The listing builds one solid part. Answer for the finished solid, in the listing's coordinates (mm). Give positions to 0.01 mm unless a question says otherwise; leave off trailing zeros. Order: outer loops, then holes, each group sorted by start corner. A loop starts at its lowest first (then second) coordinate and runs counter-clockwise, first axis right, second up. Notation, with made-up numbers: (81, 44.5) -> (121, 44.5) arc R17 cw to (121, 67.5) -> close; hole circle Ø2 at (-36, -39). An arc over 180 degrees is marked (long way). Write item = value, one per line. Start each with the question number.
```python
from build123d import *

# Parameters (mm, degrees)
SALIENTE_EXTRUIR1_DEPTH = 3
CROQUIS2_W              = 3
CROQUIS2_H              = 16
CROQUIS2_H_2            = 15
SALIENTE_EXTRUIR2_DEPTH = 3


with BuildPart() as part:
    # Croquis1 → Saliente-Extruir1 (new body)
    with BuildSketch(Plane.XY):
        Polygon((111, -25), (-111, -25), (-111, -1.5), (-108, -1.5), (-108, -3), (-105, -3), (-105, 3), (-108, 3), (-108, 1.5), (-111, 1.5), (-111, 25), (111, 25), (111, 1.5), (108, 1.5), (108, 3), (105, 3), (105, -3), (108, -3), (108, -1.5), (111, -1.5), align=None)
        with BuildLine():
            Line((80, -15), (-80, -15))
            ThreePointArc((-80, -15), (-95, 0), (-80, 15))
            Line((-80, 15), (80, 15))
            ThreePointArc((80, 15), (95, 0), (80, -15))
        make_face(mode=Mode.SUBTRACT)
    extrude(amount=SALIENTE_EXTRUIR1_DEPTH)

    # Croquis2 → Saliente-Extruir2 (add)
    with BuildSketch(Plane.ZY.offset(111)):
        with Locations((1.5, 17)):
            Rectangle(CROQUIS2_W, CROQUIS2_H)
        with Locations((1.5, -17.5)):
            Rectangle(CROQUIS2_W, CROQUIS2_H_2)
    saliente_extruir2 = extrude(amount=SALIENTE_EXTRUIR2_DEPTH)

    # Simetría1: Saliente-Extruir2 across plane
    add(saliente_extruir2.mirror(Plane(origin=(0, 0, 0), x_dir=(0, 0, 1), z_dir=(1, 0, 0))))


solid = part.part
```
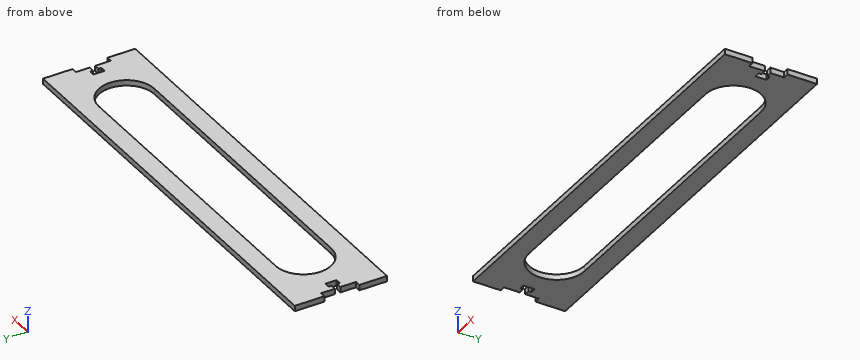
Item 1: A cutting plane is placed at B-B, the plane x = 59.5. Write down the section's boundary in (y, z).
Item 2: A cutting plane is placed at C-C, the plane y = 5.5. Write down the section's boundary in (x, z), plus the area to 3 significant figures.
Item 3: Flat-ended cylindrical pins translate along their axes: pin 1 (0.9 mm diameter, centred on y = -0.5, z = 1.5, fed in from +X); pin 2 (1.2 mm diameter, centred on y = 2.5, z = 1, fed in from -X); pin 3 (1.6 mm diameter, centred on y = 2, z = 1.5, fed in from +X); pin 4 (1.5 mm diameter, centred on x = 22, y = 12.5, fed in from +Z). Find the tip coordinate at first contact, or state that the pin passes through.
Item 4: Consider L1, parallel to Y at x = -41.5, z = 1.5; L2, parallel to X at y = 10, z = 0.45; L3, parallel to X at y = 6, z = 2. Determine where each line is inside the solid, lowest interval first. Write a range as from..to.
Check values:
q1.outline = (-25, 0) -> (-15, 0) -> (-15, 3) -> (-25, 3) -> close; (15, 0) -> (25, 0) -> (25, 3) -> (15, 3) -> close
q2.outline = (-111, 0) -> (-93.96, 0) -> (-93.96, 3) -> (-111, 3) -> close; (93.96, 0) -> (111, 0) -> (111, 3) -> (93.96, 3) -> close
q2.area = 102 mm^2
q3.pin_1 = 105
q3.pin_2 = -111
q3.pin_3 = 111
q3.pin_4 = through
q4.L1 = -25..-15, 15..25
q4.L2 = -114..-91.18, 91.18..114
q4.L3 = -111..-93.75, 93.75..111
